from build123d import *

# Parameters (mm, degrees)
BOSS_EXTRUDE1_DEPTH     = 165.1
CUT_EXTRUDE1_DEPTH      = 171.506664093
CUT_EXTRUDE1_DEPTH_BACK = 171.506664093
SKETCH2_R               = 2.5
SKETCH2_R_2             = 7.5


with BuildPart() as part:
    # Sketch1 → Boss-Extrude1 (new, symmetric)
    with BuildSketch(Plane(origin=(0, 0, 0), x_dir=(1, 0, 0), z_dir=(0, 1, 0))):
        Polygon((15.875, -19.05), (15.875, 15.875), (-19.05, 15.875), (-19.05, 19.05), (19.05, 19.05), (19.05, -19.05), align=None)
    extrude(amount=BOSS_EXTRUDE1_DEPTH, both=True)

    # Sketch2 → Cut-Extrude1 (cut, two sides: drawn at the far end of the back side and taken through both)
    with BuildSketch(Plane(origin=(19.05, 0, 0), x_dir=(0, 0, -1), z_dir=(1, 0, 0)).offset(-CUT_EXTRUDE1_DEPTH_BACK)):
        with Locations((-32.722, 128.8161)):
            Circle(SKETCH2_R)
        with Locations((-32.722, 201.3839)):
            Circle(SKETCH2_R_2)
        with Locations((-32.722, -17.2339)):
            Circle(SKETCH2_R)
        with Locations((-32.722, -70.5739)):
            Circle(SKETCH2_R_2)
        with Locations((-0.762, -70.5739)):
            Circle(SKETCH2_R_2)
        with Locations((-0.762, 201.3839)):
            Circle(SKETCH2_R_2)
        with Locations((-0.762, 128.8161)):
            Circle(SKETCH2_R)
        with Locations((-0.762, -17.2339)):
            Circle(SKETCH2_R)
    extrude(amount=CUT_EXTRUDE1_DEPTH + CUT_EXTRUDE1_DEPTH_BACK, mode=Mode.SUBTRACT)


solid = part.part
The model under review builds one solid part; all positions refer to its coordinate system, in mm. A direction names the side the tool comes from. Round coordinates to 2 decimals unless told otherwise and drop trailing zeros. Order: outer loops, then holes, each group sorted by start corner. A loop starts at its lowest first (then second) coordinate and runs counter-clockwise, first axis right, second up. Notation, with made-up numbers: (65.25, 63) - (112.25, 63) arc R21 ccw to (112.25, 99) - close; hole circle Ø2 at (76, 68.25). An arc over 180 degrees is marked (long way). Use one line per item in the form item = value.
Q1. Clearance check with flat-ended pins moving along their axes: P1, Ø17.5, axis at x = 3.5, y = -23.5, coming from the +Z side (3 decimals); P2, Ø12, axis at x = -6, z = -6, coming from the -Y side; P3, Ø6.5, axis at y = 128.82, z = 0.76, coming from the -X side (3 decimals). State where each tip first meets the part, or that it passes through.
Response values:
P1 = -15.875
P2 = through
P3 = 15.875
Q2. Add section B-B on y = 0. Give the boundary of the cut face in (x, z) (3 decimals).
Response values:
outline = (-19.05, -19.05) - (19.05, -19.05) - (19.05, 19.05) - (15.875, 19.05) - (15.875, -15.875) - (-19.05, -15.875) - close
Q3. Tool access review of faces 1 (the flat face through (-1, 2, -15.875)), 2 (the flat face through (0, 2, -19.05)): name each direction out of +Z, -Z, +X, -X, +Y, -Y from which nothing blocks a thin tool from reaching the whole face with its end or side.
Response values:
face_1 = +Z, -X, +Y, -Y
face_2 = -Z, +X, -X, +Y, -Y
Q4. Add section A-A on x = 2.5. Give the boundary of the cut face in (y, z) (3 decimals).
Response values:
outline = (-165.1, -19.05) - (165.1, -19.05) - (165.1, -15.875) - (-165.1, -15.875) - close
Q5. Mouldability with a two-part tool opening along Y and no side actions: class faces 3 (the flat face through (15.875, 2, 2)), 4 (the flat face through (17, -165.1, -9)), 5 (the flat face through (17, 165.1, -9)), 6 (the cylindrical face through (17.44, -63.138, 1.738)) as pulls with the +Y half, pulls with the -Y half, needs draft (parallel to the pull), parting line crosses it, or undercut.
Response values:
face_3 = needs draft
face_4 = pulls with the -Y half
face_5 = pulls with the +Y half
face_6 = undercut
Q6. To check wall thickness, follow line 1 (X direction, y = -56.5, z = -9) (3 decimals); line 2 (Z direction, x = 10, y = -85.5) (3 decimals). State the ranges of each line that lie inside material, in increasing order.
Response values:
line_1 = 15.875 to 19.05
line_2 = -19.05 to -15.875
